```python
from build123d import *

# Parameters (mm, degrees)
SKETCH1_W           = 68.5
SKETCH1_H           = 5.5
BOSS_EXTRUDE1_DEPTH = 40.75
SKETCH2_W           = 68.5
SKETCH2_H           = 2.25
CUT_EXTRUDE1_DEPTH  = 3


with BuildPart() as part:
    # Sketch1 → Boss-Extrude1 (new, symmetric)
    with BuildSketch(Plane.XY):
        Rectangle(SKETCH1_W, SKETCH1_H)
    extrude(amount=BOSS_EXTRUDE1_DEPTH, both=True)

    # Sketch2 → Cut-Extrude1 (cut)
    with BuildSketch(Plane.XY.offset(40.75)):
        with Locations((0, 1.625)):
            Rectangle(SKETCH2_W, SKETCH2_H)
        with Locations((0, -1.625)):
            Rectangle(SKETCH2_W, SKETCH2_H)
    extrude(amount=-CUT_EXTRUDE1_DEPTH, mode=Mode.SUBTRACT)


solid = part.part
```
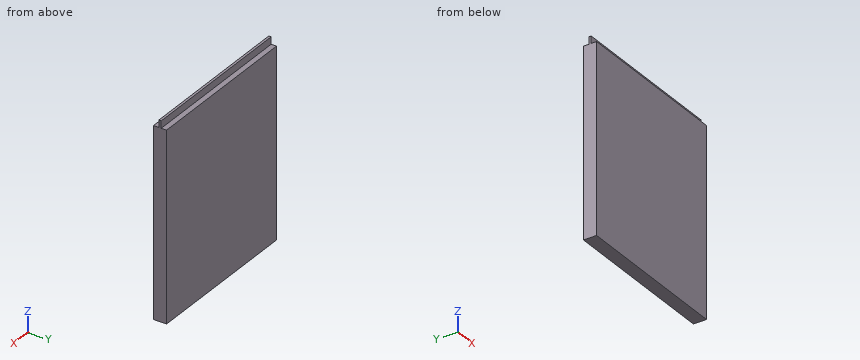
Can you work these out from the model? Positions are in its coordinate system, mm. Round coordinates to 2 decimals unless told otherwise and drop trailing zeros. Loops run counter-clockwise (first coordinate to the right, second up) from the corner with the lowest first, then second, coordinate; pieces in that order, holes last. Notation, with made-up numbers: M -20.75,51 L 3.25,51 A34 ccw 3.25,86 Z; hole C 66.5,-10.75 d11. An arc over 180 degrees is marked long. Write item = value, one per line. Start each with the question number.
(1) I need wall thicknesses on line 1 along Z through (x, y) = (15.5, 1.75). Which ranges of the line are inside material? Lowest first, please.
(2) Suppose I cut it at A-A on x = -2.5. Write out the boundary of the cut face in (y, z).
(3) I'm going to push flat-ended pins straight in: P1, Ø2.5, axis at x = 0.5, y = -2, coming from the +Z side; P2, Ø0.9, axis at x = -5, z = 38.5, coming from the -Y side; P3, Ø0.9, axis at x = -0.5, z = 39, coming from the +Y side. Where does each tip first touch, or does it pass through?
(4) Suppose I cut it at B-B on y = 1.7. Write out the boundary of the cut face in (x, z), plus the area to 3 significant figures.
Answer block:
q1.line_1 = -40.75 to 37.75
q2.outline = M -2.75,-40.75 L 2.75,-40.75 L 2.75,37.75 L 0.5,37.75 L 0.5,40.75 L -0.5,40.75 L -0.5,37.75 L -2.75,37.75 Z
q3.P1 = 37.75
q3.P2 = -0.5
q3.P3 = 0.5
q4.outline = M -34.25,-40.75 L 34.25,-40.75 L 34.25,37.75 L -34.25,37.75 Z
q4.area = 5,380 mm²
